Design review of the part built by this model. Coordinates are the model's own, in mm. Give positions to 0.01 mm unless a question says otherwise; leave off trailing zeros. Loops run counter-clockwise (first coordinate to the right, second up) from the corner with the lowest first, then second, coordinate; pieces in that order, holes last. Notation, with made-up numbers: (-6.5, 49) -> (13.5, 49) arc R20 ccw to (13.5, 67) -> close; hole circle Ø8 at (76.25, 76.25). An arc over 180 degrees is marked (long way). Answer in a Markdown table with one row per item. Add a question column.
(1) For pin 1 (2 mm diameter, centred on x = 17, z = 3, fed in from -Y); pin 2 (2 mm diameter, centred on x = 34.925, y = 22.225, fed in from +Z), all flat-tipped, find the tip position at first contact; note any pin that passes through.
(2) Consider section A-A on y = 6. Write out the cut boundary in (x, z).
(3) Consider section B-B on x = 0.5. Write out the cut boundary in (y, z), then the cut area to 3 significant figures.
(4) Consider section C-C on z = 2.25. Write out the cut boundary in (x, y) (3 decimals), then the cut area to 3 significant figures.
(5) For line 1 (Y direction, x = 7, z = 0.95); line 2 (X direction, y = -22, z = 0.75); line 3 (X direction, y = -5.5, z = 0.3), list the stretches that pass through material, from the lowest coordinate up.
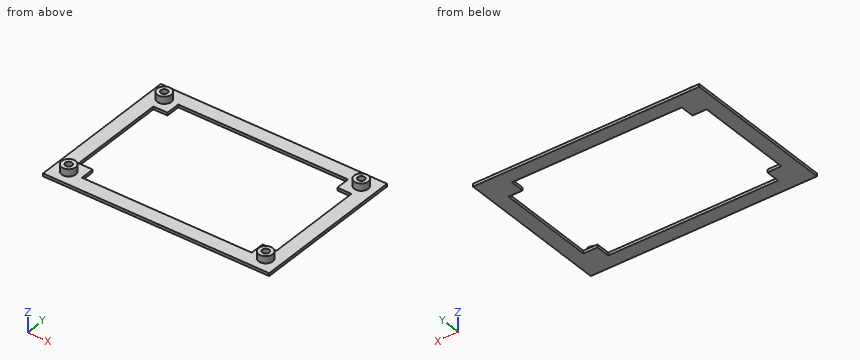
from build123d import *

# Parameters (mm, degrees)
SKETCH_W        = 80.2
SKETCH_H        = 54.8
PAD_DEPTH       = 1
POCKET_DEPTH    = 1.001
SKETCH002_R     = 2.5
PAD001_DEPTH    = 2.5
SKETCH003_R     = 1.2
POCKET001_DEPTH = 2.5


with BuildPart() as part:
    # Sketch → Pad (new body)
    with BuildSketch(Plane.XY):
        Rectangle(SKETCH_W, SKETCH_H)
    extrude(amount=PAD_DEPTH)

    # Sketch001 → Pocket (cut, through all)
    with BuildSketch(Plane.XY.offset(1)):
        Polygon((-35.1, 17.4), (-35.1, -17.4), (-30.1, -17.4), (-30.1, -22.4), (30.1, -22.4), (30.1, -17.4), (35.1, -17.4), (35.1, 17.4), (30.1, 17.4), (30.1, 22.4), (-30.1, 22.4), (-30.1, 17.4), align=None)
    extrude(amount=-POCKET_DEPTH, mode=Mode.SUBTRACT)

    # Sketch002 → Pad001 (new body)
    with BuildSketch(Plane.XY.offset(1)):
        with Locations((-34.925, 22.225)):
            Circle(SKETCH002_R)
        with Locations((-34.925, -22.225)):
            Circle(SKETCH002_R)
        with Locations((34.925, 22.225)):
            Circle(SKETCH002_R)
        with Locations((34.925, -22.225)):
            Circle(SKETCH002_R)
    extrude(amount=PAD001_DEPTH)

    # Sketch003 → Pocket001 (cut)
    with BuildSketch(Plane.XY.offset(3.5)):
        with Locations((-34.925, -22.225)):
            Circle(SKETCH003_R)
        with Locations((34.925, -22.225)):
            Circle(SKETCH003_R)
        with Locations((-34.925, 22.225)):
            Circle(SKETCH003_R)
        with Locations((34.925, 22.225)):
            Circle(SKETCH003_R)
    extrude(amount=-POCKET001_DEPTH, mode=Mode.SUBTRACT)


solid = part.part
Values follow:
| question | item | result |
|---|---|---|
| 1 | pin 1 | through |
| 1 | pin 2 | z = 1 |
| 2 | outline | (-40.1, 0) -> (-35.1, 0) -> (-35.1, 1) -> (-40.1, 1) -> close; (35.1, 0) -> (40.1, 0) -> (40.1, 1) -> (35.1, 1) -> close |
| 3 | outline | (-27.4, 0) -> (-22.4, 0) -> (-22.4, 1) -> (-27.4, 1) -> close; (22.4, 0) -> (27.4, 0) -> (27.4, 1) -> (22.4, 1) -> close |
| 3 | area | 10.0 mm2 |
| 4 | outline | circle Ø5 at (-34.925, -22.225); circle Ø5 at (-34.925, 22.225); circle Ø5 at (34.925, -22.225); circle Ø5 at (34.925, 22.225); hole circle Ø2.4 at (-34.925, -22.225); hole circle Ø2.4 at (-34.925, 22.225); hole circle Ø2.4 at (34.925, -22.225); hole circle Ø2.4 at (34.925, 22.225) |
| 4 | area | 60.4 mm2 |
| 5 | line 1 | -27.4 to -22.4, 22.4 to 27.4 |
| 5 | line 2 | -40.1 to -30.1, 30.1 to 40.1 |
| 5 | line 3 | -40.1 to -35.1, 35.1 to 40.1 |
